Can you work these out from the model? Positions are in its coordinate system, mm. Coordinates: 2 decimals unless noted, no trailing zeros. Answer in a Markdown table with one row per item.
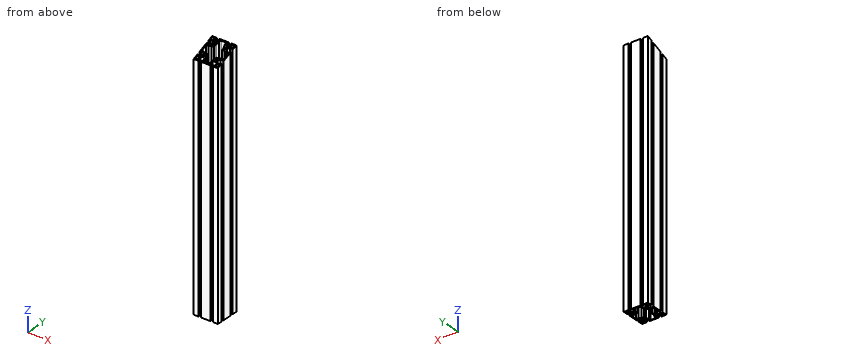
```python
from build123d import *

# Parameters (mm, degrees)
F0_R          = 3
F0_R_2        = 2.5
F1_DEPTH      = 610
F2_R          = 2
F3_R          = 7
F5_DEPTH      = 30
F5_DEPTH_BACK = 30


# Not quite as in the source:
# - a feature names something its author has since deleted; it is built from what else it names


with BuildPart() as f1:
    # F0 (on Top) → F1 (new body)
    with BuildSketch(Plane.XY):
        with BuildLine():
            Line((18.15, -30), (30, -30))
            Line((30, -30), (30, -18.15))
            Line((30, -18.15), (27.5, -18.15))
            Line((27.5, -18.15), (27.5, -20.15))
            Line((27.5, -20.15), (21.5477069044, -20.15))
            ThreePointArc((21.5477069044, -20.15), (19.5, -15), (21.5477069044, -9.85))
            Line((21.5477069044, -9.85), (27.5, -9.85))
            Line((27.5, -9.85), (27.5, -11.85))
            Line((27.5, -11.85), (30, -11.85))
            Line((30, -11.85), (30, 11.85))
            Line((30, 11.85), (27.5, 11.85))
            Line((27.5, 11.85), (27.5, 9.85))
            Line((27.5, 9.85), (21.5477069044, 9.85))
            ThreePointArc((21.5477069044, 9.85), (19.5, 15), (21.5477069044, 20.15))
            Line((21.5477069044, 20.15), (27.5, 20.15))
            Line((27.5, 20.15), (27.5, 18.15))
            Line((27.5, 18.15), (30, 18.15))
            Line((30, 18.15), (30, 30))
            Line((30, 30), (18.15, 30))
            Line((18.15, 30), (18.15, 27.5))
            Line((18.15, 27.5), (20.15, 27.5))
            Line((20.15, 27.5), (20.15, 21.5477069044))
            ThreePointArc((20.15, 21.5477069044), (15, 19.5), (9.85, 21.5477069044))
            Line((9.85, 21.5477069044), (9.85, 27.5))
            Line((9.85, 27.5), (11.85, 27.5))
            Line((11.85, 27.5), (11.85, 30))
            Line((11.85, 30), (-11.85, 30))
            Line((-11.85, 30), (-11.85, 27.5))
            Line((-11.85, 27.5), (-9.85, 27.5))
            Line((-9.85, 27.5), (-9.85, 21.5477069044))
            ThreePointArc((-9.85, 21.5477069044), (-15, 19.5), (-20.15, 21.5477069044))
            Line((-20.15, 21.5477069044), (-20.15, 27.5))
            Line((-20.15, 27.5), (-18.15, 27.5))
            Line((-18.15, 27.5), (-18.15, 30))
            Line((-18.15, 30), (-30, 30))
            Line((-30, 30), (-30, 18.15))
            Line((-30, 18.15), (-27.5, 18.15))
            Line((-27.5, 18.15), (-27.5, 20.15))
            Line((-27.5, 20.15), (-21.5477069044, 20.15))
            ThreePointArc((-21.5477069044, 20.15), (-19.5, 15), (-21.5477069044, 9.85))
            Line((-21.5477069044, 9.85), (-27.5, 9.85))
            Line((-27.5, 9.85), (-27.5, 11.85))
            Line((-27.5, 11.85), (-30, 11.85))
            Line((-30, 11.85), (-30, -11.85))
            Line((-30, -11.85), (-27.5, -11.85))
            Line((-27.5, -11.85), (-27.5, -9.85))
            Line((-27.5, -9.85), (-21.5477069044, -9.85))
            ThreePointArc((-21.5477069044, -9.85), (-19.5, -15), (-21.5477069044, -20.15))
            Line((-21.5477069044, -20.15), (-27.5, -20.15))
            Line((-27.5, -20.15), (-27.5, -18.15))
            Line((-27.5, -18.15), (-30, -18.15))
            Line((-30, -18.15), (-30, -30))
            Line((-30, -30), (-18.15, -30))
            Line((-18.15, -30), (-18.15, -27.5))
            Line((-18.15, -27.5), (-20.15, -27.5))
            Line((-20.15, -27.5), (-20.15, -21.5477069044))
            ThreePointArc((-20.15, -21.5477069044), (-15, -19.5), (-9.85, -21.5477069044))
            Line((-9.85, -21.5477069044), (-9.85, -27.5))
            Line((-9.85, -27.5), (-11.85, -27.5))
            Line((-11.85, -27.5), (-11.85, -30))
            Line((-11.85, -30), (11.85, -30))
            Line((11.85, -30), (11.85, -27.5))
            Line((11.85, -27.5), (9.85, -27.5))
            Line((9.85, -27.5), (9.85, -21.5477069044))
            ThreePointArc((9.85, -21.5477069044), (15, -19.5), (20.15, -21.5477069044))
            Line((20.15, -21.5477069044), (20.15, -27.5))
            Line((20.15, -27.5), (18.15, -27.5))
            Line((18.15, -27.5), (18.15, -30))
        make_face()
        with Locations((-25, -25)):
            Circle(F0_R, mode=Mode.SUBTRACT)
        with Locations((-15, -15)):
            Circle(F0_R_2, mode=Mode.SUBTRACT)
        with Locations((25, -25)):
            Circle(F0_R, mode=Mode.SUBTRACT)
        with Locations((15, -15)):
            Circle(F0_R_2, mode=Mode.SUBTRACT)
        with Locations((-25, 25)):
            Circle(F0_R, mode=Mode.SUBTRACT)
        with Locations((-15, 15)):
            Circle(F0_R_2, mode=Mode.SUBTRACT)
        Polygon((-7, 22), (-7, 27.5), (0, 27.5), (7, 27.5), (7, 22), (10, 16), (10, 10), (16, 10), (22, 7), (27.5, 7), (27.5, 0), (27.5, -7), (22, -7), (16, -10), (10, -10), (10, -16), (7, -22), (7, -27.5), (0, -27.5), (-7, -27.5), (-7, -22), (-10, -16), (-10, -10), (-16, -10), (-22, -7), (-27.5, -7), (-27.5, 0), (-27.5, 7), (-22, 7), (-16, 10), (-10, 10), (-10, 16), align=None, mode=Mode.SUBTRACT)
        with Locations((15, 15)):
            Circle(F0_R_2, mode=Mode.SUBTRACT)
        with Locations((25, 25)):
            Circle(F0_R, mode=Mode.SUBTRACT)
    extrude(amount=F1_DEPTH)

    # F2
    f2_edges = [f1.edges().sort_by_distance(p)[0] for p in [
        (-7, 27.5, 305),
        (7, 27.5, 305),
    ]]
    fillet(f2_edges, radius=F2_R)

    # F3
    f3_edges = [f1.edges().sort_by_distance(p)[0] for p in [
        (-10, 16, 305),
        (10, 16, 305),
    ]]
    fillet(f3_edges, radius=F3_R)

    # F4 (on Right) → F5 (cut, two sides)
    with BuildSketch(Plane.YZ) as f5_sk:
        Polygon((-66.9285170742, 844.0061405012), (-249.6042822322, 768.3393610558), (-152.6757651581, 534.3332205546), (30, 610), align=None)
    extrude(amount=F5_DEPTH, mode=Mode.SUBTRACT)
    extrude(f5_sk.sketch, amount=-F5_DEPTH_BACK, mode=Mode.SUBTRACT)


solid = f1.part
```
(1) Will these pins go through, and if not, where does the flat tip stop? pin 1 Ø3 at (x, y) = (-8, 11.5) entering from -Z; pin 2 Ø6 at (y, z) = (18, 306.5) entering from +X.
Response values:
| item | result |
|---|---|
| pin 1 | through |
| pin 2 | x = 30 |
(2) I need wall thicknesses on line 1 (Y direction, x = 15, z = 342); line 2 (Y direction, x = -25, z = 123); line 3 (X direction, y = 24.5, z = 278). Which ranges of each line are inside material? Lowest first, please. Write a range as [from, to].
Response values:
| item | result |
|---|---|
| line 1 | [-19.5, -17.5], [-12.5, -10], [10, 12.5], [17.5, 19.5] |
| line 2 | [-30, -28], [-22, -20.15], [-9.85, -7], [7, 9.85], [20.15, 22], [28, 30] |
| line 3 | [-30, -27.96], [-22.04, -20.15], [-9.85, -7], [7, 9.85], [20.15, 22.04], [27.96, 30] |
(3) Suppose I cut it at A-A (z = 144). Count the separate pieces of the cut face and the enclosed holes in it, and give its area (3 significant figures).
Response values:
| item | result |
|---|---|
| separate pieces | 1 |
| enclosed holes | 9 |
| area | 1,080 mm2 |
